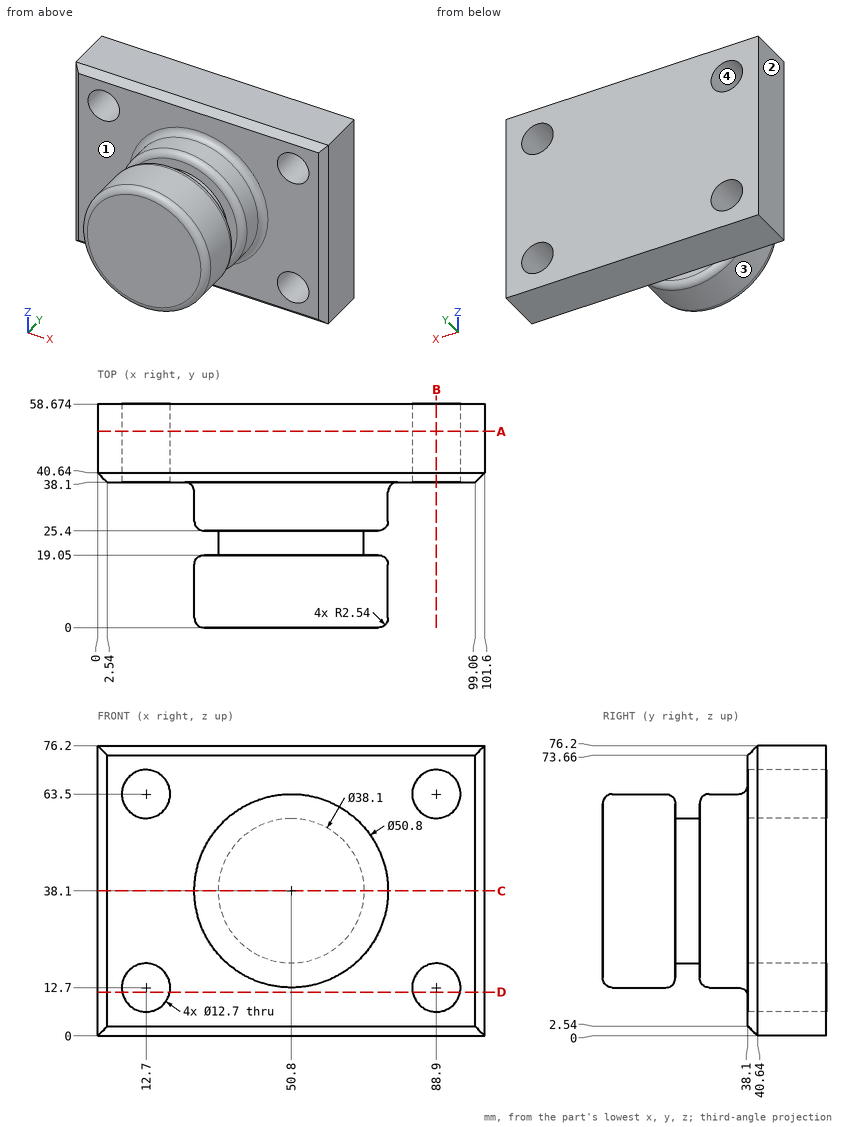
Design review of the part shown in the three views and the two pictorial views. Dimensions are in mm from the part's minimum x, y and z. Round coordinates to 2 decimals unless told otherwise and drop trailing zeros. Write each loop counter-clockwise with the first axis right and the second up, starting at its lowest first coordinate (ties: lowest second). Pieces come first, ordered by that corner, then holes. Notation, with made-up numbers: (-15, 6.25) -> (-6, 6.25) arc R21 ccw to (-6, 13.25) -> close; hole circle Ø3 at (81.25, 11). An arc over 180 degrees is marked (long way). Write item = value, one per line. Start each with the question number.
1) Clearance check with flat-ended pins moving along their axes: pin 1 (10 mm diameter, centred on x = 41, y = 16, fed in from +Z); pin 2 (14.5 mm diameter, centred on x = 12.7, z = 63.5, fed in from -Y); pin 3 (6 mm diameter, centred on y = 17, z = 28.5, fed in from +X). State where each tip first meets the part, or that it passes through.
2) Take a section at D-D, the plane z = 11.5. Count the separate pieces of the cut face and the enclosed holes in it, plus the area to 3 significant figures.
3) Take a section at A-A, the plane y = 51.5. State the section outline as (x, z) points, plus the area to 3 significant figures.
4) Mouldability with a two-part tool opening along X and no side actions: class the marked faces 1, 2, 3 and 4 as +X half, -X half, draft (parallel to the pull), parting line (faces both ways), or undercut.
5) Take a section at C-C, the plane z = 38.1. State the section outline as (x, y) points.
6) Wall thickness on probe 1 along Z at (x, y) = (88.9, 46.25); probe 2 along X at (y, z) = (53, 63); probe 3 along Y at (x, z) = (72, 32): over which ranges is each line inside the solid? List them lowest first. Write a range as from..to.
7) Take a section at B-B, the plane x = 88.9. State the section outline as (y, z) points.
Results list:
q1.pin_1 = 63.04
q1.pin_2 = 38.1
q1.pin_3 = 75.32
q2.separate_pieces = 3
q2.enclosed_holes = 0
q2.area = 1,570 mm²
q3.outline = (0, 0) -> (101.6, 0) -> (101.6, 76.2) -> (0, 76.2) -> close; hole circle Ø12.7 at (12.7, 12.7); hole circle Ø12.7 at (12.7, 63.5); hole circle Ø12.7 at (88.9, 12.7); hole circle Ø12.7 at (88.9, 63.5)
q3.area = 7,240 mm²
q4.face_1 = draft
q4.face_2 = -X half
q4.face_3 = parting line
q4.face_4 = undercut
q5.outline = (0, 40.64) -> (2.54, 38.1) -> (22.86, 38.1) arc R2.54 cw to (25.4, 35.56) -> (25.4, 27.94) arc R2.54 ccw to (27.94, 25.4) -> (31.75, 25.4) -> (31.75, 19.05) -> (27.94, 19.05) arc R2.54 ccw to (25.4, 16.51) -> (25.4, 2.54) arc R2.54 ccw to (27.94, 0) -> (73.66, 0) arc R2.54 ccw to (76.2, 2.54) -> (76.2, 16.51) arc R2.54 ccw to (73.66, 19.05) -> (69.85, 19.05) -> (69.85, 25.4) -> (73.66, 25.4) arc R2.54 ccw to (76.2, 27.94) -> (76.2, 35.56) arc R2.54 cw to (78.74, 38.1) -> (99.06, 38.1) -> (101.6, 40.64) -> (101.6, 58.67) -> (0, 58.67) -> close
q6.probe_1 = 0..6.35, 19.05..57.15, 69.85..76.2
q6.probe_2 = 0..6.37, 19.03..82.57, 95.23..101.6
q6.probe_3 = 0..19.05, 25.4..58.67
q7.outline = (38.1, 2.54) -> (40.64, 0) -> (58.67, 0) -> (58.67, 6.35) -> (38.1, 6.35) -> close; (38.1, 19.05) -> (58.67, 19.05) -> (58.67, 57.15) -> (38.1, 57.15) -> close; (38.1, 69.85) -> (58.67, 69.85) -> (58.67, 76.2) -> (40.64, 76.2) -> (38.1, 73.66) -> close
